The model under review builds one solid part; all positions refer to its coordinate system, in mm. A direction names the side the tool comes from. Round coordinates to 2 decimals unless told otherwise and drop trailing zeros. Order: outer loops, then holes, each group sorted by start corner. A loop starts at its lowest first (then second) coordinate and runs counter-clockwise, first axis right, second up.
1) Consider section A-A (x = 1.75). Give the boundary of the cut face in (y, z) (1 decimal), then the cut area to 3 significant figures.
2) Consider section D-D (x = 2.5). Give the boundary of the cut face in (y, z) (1 decimal).
3) Mouldability with a two-part tool opening along Z and no side actions: class faces 5 (the face through (3, 2, 4.366)), 6 (the face through (3, 3.175, 3)), 7 (the face through (4, 7, -2.381)), 8 (the face through (4, 12, 1.191)) as pulls with the +Z half, pulls with the -Z half, needs draft (parallel to the pull), parting line crosses it, or undercut.
4) To check wall thickness, follow L1, parallel to Z at x = 4.25, y = 1.25; L2, parallel to X at y = 3.25, z = 0; L3, parallel to Z at x = 4, y = 1.75. State the ranges of each line that lie inside material, in increasing order.
5) Machinability: for faces 1 (the face through (4, 5, 1.191)), 2 (the face through (0.201, 7.591, -2.227)), 3 (the face through (3, 6, 1.984)), 4 (the face through (5.65, 13.07, -1.63)), which of the approach directions +Z, -Z, +X, -X, +Y, -Y give a long, thin tool a straight path to every point of the face, cutting with its end or side? Answer none if there is none.
6) Consider section C-C (z = -3.75). Give the boundary of the cut face in (x, y), then the cut area to 3 significant figures.
7) Clearance check with flat-ended pins moving along their axes: P1, Ø3, axis at x = 3, y = 6, coming from the +Z side; P2, Ø4, axis at x = 3.57, y = 3.97, coming from the -Z side; P3, Ø1, axis at x = 3, z = 0.5, coming from the +Y side. State where each tip first meets the part, or that it passes through.
from build123d import *

# Parameters (mm, degrees)
BOSS_EXTRUDE4_DEPTH  = 6.746875
SKETCH6_R            = 3.96875
BOSS_EXTRUDE5_DEPTH  = 6.746875
SHELL2_T             = -0.79375
BOSS_EXTRUDE6_REACH  = 19.089
CUT_EXTRUDE2_START   = -0.396875
SKETCH11_R           = 3.96875
CUT_EXTRUDE2_DEPTH   = 0.396875
SKETCH13_R           = 3.96875
BOSS_EXTRUDE11_DEPTH = 6.35
SKETCH14_R           = 2.38125
CUT_EXTRUDE3_DEPTH   = 1.984375
CUT_EXTRUDE4_DEPTH   = 3.571875
SKETCH17_R           = 1.190625
CUT_EXTRUDE5_DEPTH   = 2.38125


with BuildPart() as part:
    # Sketch2 → Boss-Extrude4 (new body)
    with BuildSketch(Plane(origin=(0, 0, 0), x_dir=(0, 0, -1), z_dir=(1, 0, 0))):
        Polygon((-4.365625, 0), (4.365625, 0), (4.365625, 11.1125), (-1.984375, 11.1125), (-1.984375, 3.175), (-4.365625, 3.175), align=None)
    extrude(amount=BOSS_EXTRUDE4_DEPTH)

    # Sketch6 → Boss-Extrude5 (add)
    with BuildSketch(Plane(origin=(6.746875, 0, 0), x_dir=(0, 0, -1), z_dir=(1, 0, 0))):
        with Locations((0.396875, 11.1125)):
            Circle(SKETCH6_R)
    extrude(amount=-BOSS_EXTRUDE5_DEPTH)

    # Shell2
    shell2_openings = [part.faces().sort_by_distance(p)[0] for p in [
        (3.3734375, 0, 0),
    ]]
    offset(amount=SHELL2_T, openings=shell2_openings, kind=Kind.INTERSECTION)

    # Sketch7 → Boss-Extrude6 (add, up to next)
    with BuildSketch(Plane.XZ, mode=Mode.PRIVATE) as boss_extrude6_sk1:
        Polygon((5.953125, 3.571875), (5.953125, 2.38125), (1.190625, 2.38125), (1.190625, -2.38125), (5.953125, -2.38125), (5.953125, -3.571875), (0.79375, -3.571875), (0.79375, 3.571875), align=None)
    boss_extrude6_tool1 = extrude(boss_extrude6_sk1.sketch, amount=-BOSS_EXTRUDE6_REACH, mode=Mode.PRIVATE) - part.part
    add(boss_extrude6_tool1.solids().sort_by_distance((5.865004, 0, 2.976562))[0])

    # Sketch11 → Cut-Extrude2 (cut)
    with BuildSketch(Plane.ZY.offset(CUT_EXTRUDE2_START)):
        with Locations((-0.396875, 11.1125)):
            Circle(SKETCH11_R)
    extrude(amount=CUT_EXTRUDE2_DEPTH, mode=Mode.SUBTRACT)

    # Sketch13 → Boss-Extrude11 (add)
    with BuildSketch(Plane(origin=(6.746875, 0, 0), x_dir=(0, 0, -1), z_dir=(1, 0, 0))):
        with Locations((0.396875, 11.1125)):
            Circle(SKETCH13_R)
    extrude(amount=-BOSS_EXTRUDE11_DEPTH)

    # Sketch14 → Cut-Extrude3 (cut)
    with BuildSketch(Plane(origin=(0, 0, -4.365625), x_dir=(-1, 0, 0), z_dir=(0, 0, -1))):
        with Locations(Location((-3.571875, 3.96875, 0), (0, 0, 90))):
            Circle(SKETCH14_R)
        with Locations(Location((-3.571875, 11.90625, 0), (0, 0, 180))):
            Circle(SKETCH14_R)
    extrude(amount=-CUT_EXTRUDE3_DEPTH, mode=Mode.SUBTRACT)

    # Sketch16 → Cut-Extrude4 (cut)
    with BuildSketch(Plane(origin=(0, 0, -2.38125), x_dir=(-1, 0, 0), z_dir=(0, 0, -1))):
        with BuildLine():
            Line((-2.778125, 9.66118597), (-2.778125, 14.15131403))
            ThreePointArc((-2.778125, 14.15131403), (-5.953125, 11.90625), (-2.778125, 9.66118597))
        make_face()
    extrude(amount=-CUT_EXTRUDE4_DEPTH, mode=Mode.SUBTRACT)

    # Sketch17 → Cut-Extrude5 (cut)
    with BuildSketch(Plane.ZY.offset(-0.396875)):
        with Locations((-0.396875, 11.1125)):
            Circle(SKETCH17_R)
    extrude(amount=-CUT_EXTRUDE5_DEPTH, mode=Mode.SUBTRACT)


solid = part.part
Answer below:
1. outline: (0, -4.4) - (2.4, -4.4) - (2.4, -2.4) - (0, -2.4) - close; (0, 2.4) - (2.4, 2.4) - (2.4, 1.2) - (7.5, 1.2) arc R4 ccw to (7.7, -2.4) - (5.5, -2.4) - (5.5, -4.4) - (10.4, -4.4) - (10.4, -2.4) - (13.4, -2.4) - (13.4, -3.6) arc R4 ccw (long way) to (7.9, 2) - (3.2, 2) - (3.2, 4.4) - (0, 4.4) - close; hole circle Ø2.4 at (11.1, -0.4)
1. area: 61.5 mm2
2. outline: (0, -4.4) - (1.8, -4.4) - (1.8, -2.4) - (0, -2.4) - close; (0, 2.4) - (2.4, 2.4) - (2.4, 1.2) - (7.5, 1.2) arc R4 ccw to (7.7, -2.4) - (6.1, -2.4) - (6.1, -4.4) - (9.8, -4.4) - (9.8, -2.4) - (14, -2.4) - (14, -3.1) arc R4 ccw (long way) to (7.9, 2) - (3.2, 2) - (3.2, 4.4) - (0, 4.4) - close; hole circle Ø2.4 at (11.1, -0.4)
3. face 5: pulls with the +Z half
3. face 6: needs draft
3. face 7: undercut
3. face 8: pulls with the -Z half
4. L1: z = -4.37 to -2.38, 2.38 to 4.37
4. L2: x = 0 to 1.19, 5.95 to 6.75
4. L3: z = 2.38 to 4.37
5. face 1: -Y
5. face 2: -X, +Y
5. face 3: +Z, +X, -X
5. face 4: -Z
6. outline: (0, 0) - (6.75, 0) - (6.75, 13.24) - (5.55, 13.24) arc R2.38 cw (long way) to (1.6, 13.24) - (0.4, 13.24) - (0.4, 8.99) - (0, 8.99) - close; hole circle Ø4.76 at (3.57, 3.97)
6. area: 54.9 mm2
7. P1: stops at z = 1.98
7. P2: stops at z = 1.19
7. P3: stops at y = 15.06
